```python
from build123d import *

# Parameters (mm, degrees)
SKETCH1_W           = 5.35
SKETCH1_H           = 6.1
SKETCH1_W_2         = 1.35
SKETCH1_H_2         = 2.1
BOSS_EXTRUDE1_DEPTH = 6
SKETCH2_W           = 5.35
SKETCH2_H           = 6.1
BOSS_EXTRUDE2_DEPTH = 10
FILLET1_R           = 1.5
FILLET2_R           = 1.5


with BuildPart() as part:
    # Sketch1 → Boss-Extrude1 (new body)
    with BuildSketch(Plane(origin=(0, 0, 0), x_dir=(1, 0, 0), z_dir=(0, 1, 0))):
        Rectangle(SKETCH1_W, SKETCH1_H)
        Rectangle(SKETCH1_W_2, SKETCH1_H_2, mode=Mode.SUBTRACT)
    extrude(amount=BOSS_EXTRUDE1_DEPTH)

    # Sketch2 → Boss-Extrude2 (add)
    with BuildSketch(Plane(origin=(0, 6, 0), x_dir=(1, 0, 0), z_dir=(0, 1, 0))):
        Rectangle(SKETCH2_W, SKETCH2_H)
    extrude(amount=BOSS_EXTRUDE2_DEPTH)

    # Fillet1
    fillet1_edges = [part.edges().sort_by_distance(p)[0] for p in [
        (0, 0, -3.05),
        (2.675, 0, 0),
        (0, 0, 3.05),
        (-2.675, 0, 0),
    ]]
    fillet(fillet1_edges, radius=FILLET1_R)

    # Fillet2
    # the kernel refuses this fillet: 1.5 mm, written as the material it takes off along each edge
    with BuildSketch(Plane(origin=(1.175, 1.5, -1.55), x_dir=(1, 0, 0), z_dir=(0, 0, -1))) as fillet2_piece_1_section:
        Polygon((0, 0), (FILLET2_R, 0), (FILLET2_R, FILLET2_R), (0, FILLET2_R), align=None)
    fillet2_piece_1 = extrude(amount=FILLET2_R, mode=Mode.PRIVATE)
    fillet2_piece_1 = fillet2_piece_1 - Plane(origin=(1.175, 1.5, -1.55), x_dir=(-0.7071067811865475, 0.7071067811865475, 0), z_dir=(0, 0, -1)) * Sphere(FILLET2_R, mode=Mode.PRIVATE)
    add(fillet2_piece_1, mode=Mode.SUBTRACT)
    with BuildSketch(Plane(origin=(1.175, 1.5, 1.55), x_dir=(0, 0, 1), z_dir=(1, 0, 0))) as fillet2_piece_2_section:
        Polygon((0, 0), (FILLET2_R, 0), (FILLET2_R, FILLET2_R), (0, FILLET2_R), align=None)
    fillet2_piece_2 = extrude(amount=FILLET2_R, mode=Mode.PRIVATE)
    fillet2_piece_2 = fillet2_piece_2 - Plane(origin=(1.175, 1.5, 1.55), x_dir=(0, 0.7071067811865475, -0.7071067811865475), z_dir=(1, 0, 0)) * Sphere(FILLET2_R, mode=Mode.PRIVATE)
    add(fillet2_piece_2, mode=Mode.SUBTRACT)
    with BuildSketch(Plane(origin=(-1.175, 1.5, -1.55), x_dir=(-1, 0, 0), z_dir=(0, 0, -1))) as fillet2_piece_3_section:
        Polygon((0, 0), (FILLET2_R, 0), (FILLET2_R, -FILLET2_R), (0, -FILLET2_R), align=None)
    fillet2_piece_3 = extrude(amount=FILLET2_R, mode=Mode.PRIVATE)
    fillet2_piece_3 = fillet2_piece_3 - Plane(origin=(-1.175, 1.5, -1.55), x_dir=(0.7071067811865475, 0.7071067811865475, 0), z_dir=(0, 0, -1)) * Sphere(FILLET2_R, mode=Mode.PRIVATE)
    add(fillet2_piece_3, mode=Mode.SUBTRACT)
    with BuildSketch(Plane(origin=(-1.175, 1.5, 1.55), x_dir=(0, 0, 1), z_dir=(-1, 0, 0))) as fillet2_piece_4_section:
        Polygon((0, 0), (FILLET2_R, 0), (FILLET2_R, -FILLET2_R), (0, -FILLET2_R), align=None)
    fillet2_piece_4 = extrude(amount=FILLET2_R, mode=Mode.PRIVATE)
    fillet2_piece_4 = fillet2_piece_4 - Plane(origin=(-1.175, 1.5, 1.55), x_dir=(0, 0.7071067811865475, -0.7071067811865475), z_dir=(-1, 0, 0)) * Sphere(FILLET2_R, mode=Mode.PRIVATE)
    add(fillet2_piece_4, mode=Mode.SUBTRACT)
    with BuildSketch(Plane(origin=(-2.675, 1.5, -3.05), x_dir=(1, 0, 0), z_dir=(0, 1, 0)), Plane(origin=(2.675, 19.75, -3.05), x_dir=(-1, 0, 0), z_dir=(0, -1, 0)), Plane(origin=(2.675, 19.75, 3.05), x_dir=(0, 0, -1), z_dir=(0, -1, 0)), Plane(origin=(-2.675, 1.5, 3.05), x_dir=(0, 0, -1), z_dir=(0, 1, 0))) as fillet2_piece_5:
        with BuildLine():
            CenterArc((FILLET2_R, -FILLET2_R), FILLET2_R, 90, 90)
            Line((0, -FILLET2_R), (0, 0))
            Line((0, 0), (FILLET2_R, 0))
        make_face()
    extrude(amount=18.25, mode=Mode.SUBTRACT)


solid = part.part
```
Work out the finished part from the listing and answer in its coordinate system (mm). A direction names the side the tool comes from. Round coordinates to 2 decimals unless told otherwise and drop trailing zeros. Loops run counter-clockwise (first coordinate to the right, second up) from the corner with the lowest first, then second, coordinate; pieces in that order, holes last. Notation, with made-up numbers: M 45,53 L 66,53 A30 cw 66,81 Z; hole C -17,4 d4. An arc over 180 degrees is marked long. Use CSV: the item, a comma, the result in double quotes.
Q1. Section C-C, the plane y = 10.75 is taken. Determine the outline of the cut face in (x, z) (3 decimals), then the cut area to 3 significant figures.
Determined:
outline,"M -2.675,-1.55 A1.5 ccw -1.175,-3.05 L 1.175,-3.05 A1.5 ccw 2.675,-1.55 L 2.675,1.55 A1.5 ccw 1.175,3.05 L -1.175,3.05 A1.5 ccw -2.675,1.55 Z"
area,"30.7 mm2"
Q2. This flat-tipped pin is pushed along its axis until it touches: pin 1 (1.5 mm diameter, centred on x = 2, y = 5.5, fed in from +Z). Where does it stop, or does it pass through?
Determined:
pin 1,"z = 3.05"
Q3. Section D-D, the plane x = -0.3 is taken. Determine the outline of the cut face in (y, z), then the cut area to 3 significant figures.
Determined:
outline,"M 0,-1.55 A1.5 ccw 1.5,-3.05 L 16,-3.05 L 16,3.05 L 1.5,3.05 A1.5 ccw 0,1.55 L 0,1.05 L 6,1.05 L 6,-1.05 L 0,-1.05 Z"
area,"84.0 mm2"
Q4. The mould has two halves that part along X. Classify faces 1 (the flat face through (0, 9, 3.05)), 2 (the flat face through (0, 3, -1.05)), 3 (the flat face through (2.675, 9, 0)): pulls with the +X half, pulls with the -X half, needs draft (parallel to the pull), parting line crosses it, or undercut.
Determined:
face 1,"needs draft"
face 2,"undercut"
face 3,"pulls with the +X half"
Q5. A tool of negligible diameter and unlimited length cuts with its end or side. For faces 4 (the cylindrical face through (-2.247, 8.648, 2.599)), 5 (the flat face through (0, 6, 0)), from which of +Z, -Z, +X, -X, +Y, -Y can it reach the whole face along a straight path? Write none if from no direction.
Determined:
face 4,"+Z, -X, +Y, -Y"
face 5,"-Y"
Q6. Section A-A, the plane z = 0.5 is taken. Determine the outline of the cut face in (x, y) (3 decimals).
Determined:
outline,"M -2.675,1.5 A1.5 ccw -1.175,0 L -0.675,0 L -0.675,6 L 0.675,6 L 0.675,0 L 1.175,0 A1.5 ccw 2.675,1.5 L 2.675,16 L -2.675,16 Z"
Q7. Consider L1, parallel to X at y = 3.75, z = -0.75 (3 decimals); L2, parallel to X at y = 14.5, z = -2.5; L3, parallel to Y at x = 1.6, z = 0.25. Determine where each line is inside the solid, lowest interval first.
Determined:
L1,"-2.675 to -0.675, 0.675 to 2.675"
L2,"-2.34 to 2.34"
L3,"0.06 to 16"
Q8. Section B-B, the plane y = 5.5 is taken. Determine the outline of the cut face in (x, z) (3 decimals), then the cut area to 3 significant figures.
Determined:
outline,"M -2.675,-1.55 A1.5 ccw -1.175,-3.05 L 1.175,-3.05 A1.5 ccw 2.675,-1.55 L 2.675,1.55 A1.5 ccw 1.175,3.05 L -1.175,3.05 A1.5 ccw -2.675,1.55 Z; hole M -0.675,-1.05 L 0.675,-1.05 L 0.675,1.05 L -0.675,1.05 Z"
area,"27.9 mm2"
